```python
from build123d import *

# Parameters (mm, degrees)
F0_W      = 8
F0_H      = 68
F1_DEPTH  = 38
F2_SIZE   = 4
F3_W      = 38
F3_H      = 8
F4_DEPTH  = 65
F5_W      = 8
F5_H      = 38
F6_DEPTH  = 18
F7_R      = 4
F8_R      = 4
F9_W      = 8
F9_H      = 10
F10_DEPTH = 25
F11_R     = 3.862742
F12_R     = 14
F13_DEPTH = 17
F14_R     = 10
F15_DEPTH = 100


with BuildPart() as f1:
    # F0 (on Front) → F1 (new body)
    with BuildSketch(Plane.XZ):
        Rectangle(F0_W, F0_H)
    extrude(amount=-F1_DEPTH)

    # F2
    f2_edges = [f1.edges().sort_by_distance(p)[0] for p in [
        (0, 0, 34),
        (0, 38, 34),
    ]]
    chamfer(f2_edges, length=F2_SIZE)

    # F3 (on face) → F4 (join)
    with BuildSketch(Plane.YZ.offset(4)):
        with Locations((19, -30)):
            Rectangle(F3_W, F3_H)
    extrude(amount=F4_DEPTH)

    # F5 (on face) → F6 (join)
    with BuildSketch(Plane.XY.offset(-26)):
        with Locations((28, 19)):
            Rectangle(F5_W, F5_H)
    extrude(amount=F6_DEPTH)

    # F7
    f7_edges = [f1.edges().sort_by_distance(p)[0] for p in [
        (28, 0, -8),
        (28, 38, -8),
    ]]
    fillet(f7_edges, radius=F7_R)

    # F8
    f8_edges = [f1.edges().sort_by_distance(p)[0] for p in [
        (69, 38, -30),
        (69, 0, -30),
    ]]
    fillet(f8_edges, radius=F8_R)

    # F9 (on face) → F10 (cut)
    with BuildSketch(Plane.XY.offset(-26)):
        with Locations((49, 33)):
            Rectangle(F9_W, F9_H)
        with Locations((49, 5)):
            Rectangle(F9_W, F9_H)
    extrude(amount=-F10_DEPTH, mode=Mode.SUBTRACT)

    # F11
    f11_edges = [f1.edges().sort_by_distance(p)[0] for p in [
        (45, 28, -30),
        (53, 28, -30),
        (45, 10, -30),
        (53, 10, -30),
    ]]
    fillet(f11_edges, radius=F11_R)

    # F12 (on face) → F13 (join)
    with BuildSketch(Plane.YZ.offset(4)):
        with Locations((19, 13.152632)):
            Circle(F12_R)
    extrude(amount=F13_DEPTH)

    # F14 (on face) → F15 (cut)
    with BuildSketch(Plane.YZ.offset(21)):
        with Locations((19, 13.152632)):
            Circle(F14_R)
    extrude(amount=-F15_DEPTH, mode=Mode.SUBTRACT)


solid = f1.part
```
The model under review builds one solid part; all positions refer to its coordinate system, in mm. A direction names the side the tool comes from. Give positions to 0.01 mm unless a question says otherwise; leave off trailing zeros. Loops run counter-clockwise (first coordinate to the right, second up) from the corner with the lowest first, then second, coordinate; pieces in that order, holes last. Notation, with made-up numbers: (-4, 87) - (21, 87) arc R19 ccw to (21, 117) - close; hole circle Ø3 at (28.25, -8). An arc over 180 degrees is marked (long way). Answer as a JSON object with one key per item and string values.
Q1. For faces 4 (the flat face through (28, 19, -8)), 5 (the flat face through (24, 19, -17)), 6 (the flat face through (45, 3, -30)), 7 (the cylindrical face through (12.381, 31.932, 7.791)), 8 (the flat face through (53, 35, -30)), list the 3-axis set-ups (+Z, -Z, +X, -X, +Y, -Y) from which the entire face can be reached by the end or side of a thin tool; tool diameter is ignored.
Worked out:
{"face 4": "+Z, +X, +Y, -Y", "face 5": "+Z, +Y, -Y", "face 6": "+Z, -Z, -Y", "face 7": "+X", "face 8": "+Z, -Z, +Y"}
Q2. Add section B-B on y = 19. State the section outline as (x, z) points.
Worked out:
{"outline": "(-4, -34) - (69, -34) - (69, -26) - (32, -26) - (32, -8) - (24, -8) - (24, -26) - (4, -26) - (4, -0.85) - (21, -0.85) - (21, 3.15) - (-4, 3.15) - close; (-4, 23.15) - (21, 23.15) - (21, 27.15) - (4, 27.15) - (4, 34) - (-4, 34) - close"}
Q3. Add section A-A on z = -16. State the section outline as (x, y) points, plus the area to 3 significant figures.
Worked out:
{"outline": "(-4, 0) - (4, 0) - (4, 38) - (-4, 38) - close; (24, 0) - (32, 0) - (32, 38) - (24, 38) - close", "area": "608 mm^2"}
Q4. Add section D-D on x = 42. State the section outline as (y, z) points.
Worked out:
{"outline": "(0, -34) - (38, -34) - (38, -26) - (0, -26) - close"}
Q5. Add section C-C on x = 18.5. State the section outline as (y, z) points.
Worked out:
{"outline": "(0, -34) - (38, -34) - (38, -26) - (0, -26) - close; circle Ø28 at (19, 13.15); hole circle Ø20 at (19, 13.15)"}
Q6. Mouldability with a two-part tool opening along Z and no side actions: class faces 1 (the flat face through (45, 35, -30)), 2 (the cylindrical face through (8.675, 28.538, 16.156)), 3 (the flat face through (32, 19, -34)) as +Z half, -Z half, draft (parallel to the pull), parting line (faces both ways), or undercut.
Worked out:
{"face 1": "draft", "face 2": "undercut", "face 3": "-Z half"}
Q7. To check wall thickness, follow line 1 along Z through (x, y) = (5.5, 19); line 2 along Z through (x, y) = (8, 12); line 3 along Z through (x, y) = (23.5, 29). State the ranges of each line that lie inside material, in increasing order.
Worked out:
{"line 1": "z = -34 to -26, -0.85 to 3.15, 23.15 to 27.15", "line 2": "z = -34 to -26, 1.03 to 6.01, 20.29 to 25.28", "line 3": "z = -34 to -26"}
Q8. Insertion check: pin 1 (6.5 mm diameter, centred on x = 26.5, y = 21, fed in from +Z); pin 2 (2 mm diameter, centred on y = 25.5, z = -21.5, fed in from +X); pin 3 (18.5 mm diameter, centred on x = 46.5, y = 27.5, fed in from +Z); pin 4 (16 mm diameter, centred on y = 19, z = 13.15, fed in from +X). Each pin has a flat end and moves straight along its axis. Give the tip position at first contact, or say it passes through.
Worked out:
{"pin 1": "stops at z = -8", "pin 2": "stops at x = 32", "pin 3": "stops at z = -26", "pin 4": "passes through"}
